Can you work these out from the model? Positions are in its coordinate system, mm. Face numbers are marked on the shaded views. A direction names the side the tool comes from. Give positions to 0.01 mm unless a question says otherwise; leave off trailing zeros. Order: outer loops, then holes, each group sorted by start corner. A loop starts at its lowest first (then second) coordinate and runs counter-clockwise, first axis right, second up. Notation, with made-up numbers: (85.5, 66.5) -> (133.5, 66.5) arc R27 ccw to (133.5, 99.5) -> close; hole circle Ø9 at (18, 15). An arc over 180 degrees is marked (long way). Answer as CSV lines item,"result".
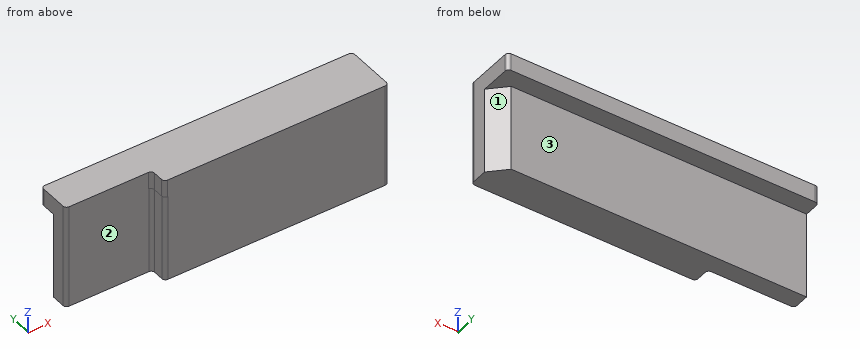
```python
from build123d import *

# Parameters (mm, degrees)
F1_DEPTH = 5
F3_DEPTH = 25


with BuildPart() as f1:
    # F0 (on Top) → F1 (new body)
    with BuildSketch(Plane.XY):
        with BuildLine():
            ThreePointArc((-32.5, -6.5), (-32.207107, -7.207107), (-31.5, -7.5))
            Line((-31.5, -7.5), (31.5, -7.5))
            ThreePointArc((31.5, -7.5), (32.207107, -7.207107), (32.5, -6.5))
            Line((32.5, -6.5), (32.5, 6.5))
            ThreePointArc((32.5, 6.5), (32.207107, 7.207107), (31.5, 7.5))
            Line((31.5, 7.5), (-32.5, 7.5))
            Line((-32.5, 7.5), (-56.5, 7.5))
            ThreePointArc((-56.5, 7.5), (-57.207107, 7.207107), (-57.5, 6.5))
            Line((-57.5, 6.5), (-57.5, -1.5))
            ThreePointArc((-57.5, -1.5), (-57.207107, -2.207107), (-56.5, -2.5))
            Line((-56.5, -2.5), (-33.5, -2.5))
            ThreePointArc((-33.5, -2.5), (-32.792893, -2.792893), (-32.5, -3.5))
            Line((-32.5, -3.5), (-32.5, -6.5))
        make_face()
    extrude(amount=F1_DEPTH)

    # F2 (on face) → F3 (join)
    with BuildSketch(Plane(origin=(0, 0, 0), x_dir=(1, 0, 0), z_dir=(0, 0, -1))):
        with BuildLine():
            Line((-57.5, 1.5), (-57.5, -2.5))
            Line((-57.5, -2.5), (27.949167, -2.5))
            Line((27.949167, -2.5), (32.5, 2))
            Line((32.5, 2), (32.5, 6.5))
            ThreePointArc((32.5, 6.5), (32.207107, 7.207107), (31.5, 7.5))
            Line((31.5, 7.5), (-31.39955, 7.5))
            ThreePointArc((-31.39955, 7.5), (-32.106657, 7.207107), (-32.39955, 6.5))
            Line((-32.39955, 6.5), (-32.39955, 3.5))
            ThreePointArc((-32.39955, 3.5), (-32.692443, 2.792893), (-33.39955, 2.5))
            Line((-33.39955, 2.5), (-33.5, 2.5))
            Line((-33.5, 2.5), (-56.5, 2.5))
            ThreePointArc((-56.5, 2.5), (-57.207107, 2.207107), (-57.5, 1.5))
        make_face()
    extrude(amount=F3_DEPTH)


solid = f1.part
```
Item 1: Please list where these lines run through material, in increasing order: line 1 along X through (y, z) = (-6.5, -21); line 2 along X through (y, z) = (-5.75, 0.75); line 3 along Y through (x, z) = (20, -3.25).
Numbers:
line 1,"x = -32.4 to 32.5"
line 2,"x = -32.5 to 32.5"
line 3,"y = -7.5 to 2.5"
Item 2: Imagine slicing it at A-A, the plane x = 14.5. Please give me the cut outline in (y, z).
Numbers:
outline,"(-7.5, -25) -> (2.5, -25) -> (2.5, 0) -> (7.5, 0) -> (7.5, 5) -> (-7.5, 5) -> close"
Item 3: For the marked faces 1, 2 and 3, which set-ups out of +Z, -Z, +X, -X, +Y, -Y let a thin tool reach every point of the face, with its end or its side?
Numbers:
face 1,"-Z, +X, +Y"
face 2,"+Z, -Z, -X, -Y"
face 3,"-Z, +X, -X, +Y"
Item 4: Imagine slicing it at C-C, the plane y = 4.5. Please give me the cut outline in (x, z), then the cut area to 3 significant figures.
Numbers:
outline,"(-57.5, 0) -> (32.5, 0) -> (32.5, 5) -> (-57.5, 5) -> close"
area,"450 mm²"
Item 5: For pin 1 (2.5 mm diameter, centred on y = -5.5, z = 3, fed in from -X); pin 2 (3.5 mm diameter, centred on y = -4.5, z = -13, fed in from -X); pin 3 (1.5 mm diameter, centred on y = 3.5, z = -5.5, fed in from +X); pin 4 (12 mm diameter, centred on x = -38, z = -5, fed in from -Y), each with a flat end and sliding along its axis, tell me the tip position at first contact or that it passes through.
Numbers:
pin 1,"stops at x = -32.5"
pin 2,"stops at x = -32.74"
pin 3,"passes through"
pin 4,"stops at y = -7.3"
Item 6: Imagine slicing it at B-B, the plane z = -18.75. Please give me the cut outline in (x, y), then the cut area to 3 significant figures.
Numbers:
outline,"(-57.5, -1.5) arc R1 ccw to (-56.5, -2.5) -> (-33.4, -2.5) arc R1 cw to (-32.4, -3.5) -> (-32.4, -6.5) arc R1 ccw to (-31.4, -7.5) -> (31.5, -7.5) arc R1 ccw to (32.5, -6.5) -> (32.5, -2) -> (27.95, 2.5) -> (-57.5, 2.5) -> close"
area,"764 mm²"
Item 7: Imagine slicing it at D-D, the plane y = 0.5. Please give me the cut outline in (x, z), then the cut area to 3 significant figures.
Numbers:
outline,"(-57.5, -25) -> (29.97, -25) -> (29.97, 0) -> (32.5, 0) -> (32.5, 5) -> (-57.5, 5) -> close"
area,"2,640 mm²"
